The listing builds one solid part. Answer for the finished solid, in the listing's coordinates (mm). Coordinates: 2 decimals unless noted, no trailing zeros. Write each loop counter-clockwise with the first axis right and the second up, starting at its lowest first coordinate (ties: lowest second). Pieces come first, ordered by that corner, then holes. Notation, with made-up numbers: M 58,70 L 113,70 A22 ccw 113,91 Z; hole C 31.5,-3 d3. An arc over 180 degrees is marked long. Answer as CSV lines item,"result".
```python
from build123d import *

# Parameters (mm, degrees)
F0_W     = 2.0093368366
F0_H     = 6.8891588598
F1_DEPTH = 25.4
F2_W     = 2.0093368366
F2_H     = 6.8161971867
F3_DEPTH = 25.4
F5_DEPTH = 25.4


with BuildPart() as f1:
    # F0 (on Front) → F1 (new body)
    with BuildSketch(Plane.XZ):
        with Locations((-14.7031224333, 14.6663570777)):
            Rectangle(F0_W, F0_H)
    extrude(amount=F1_DEPTH)

    # F2 (on face) → F3 (join)
    with BuildSketch(Plane.XZ.offset(25.4)):
        with Locations((-14.7031224333, 21.5190351009)):
            Rectangle(F2_W, F2_H)
    extrude(amount=-F3_DEPTH)

    # F4 (on face) → F5 (join)
    with BuildSketch(Plane.XZ.offset(25.4)):
        Polygon((-15.7077908516, 26.9609466195), (-15.7077908516, 24.9271336943), (-13.698454015, 24.9271336943), align=None)
        Polygon((-13.698454015, 11.2217776477), (-15.7077908516, 11.2217776477), (-15.7077908516, 9.18235071), align=None)
    extrude(amount=-F5_DEPTH)


solid = f1.part
```
Q1. Find section B-B (x = -14.8). Give the vertices of the cut face in (y, z), and give its area (3 significant figures).
Output:
outline,"M -25.4,10.1 L 0,10.1 L 0,26.04 L -25.4,26.04 Z"
area,"405 mm2"
Q2. Find section A-A (y = -11). Give the vertices of the cut face in (x, z).
Output:
outline,"M -15.71,9.18 L -13.7,11.22 L -13.7,24.93 L -15.71,26.96 Z"
Q3. Straight lines are drawn through the part: line 1 (Z direction, x = -14.25, y = -13.5); line 2 (Z direction, x = -15.6, y = -13.25); line 3 (X direction, y = -23, z = 26.25). For each, find the intervals that lie inside material, in ascending order.
Output:
line 1,"10.66 to 25.49"
line 2,"9.29 to 26.85"
line 3,"-15.71 to -15.01"
